```python
from build123d import *

# Parameters (mm, degrees)
BASE_EXTRUDE_THIN_DEPTH        = 19.05
CUT_EXTRUDE1_REACH             = 97.25
SKETCH2_R                      = 6.35
BOSS_EXTRUDE1_START            = -19.05
BOSS_EXTRUDE1_DEPTH            = 38.1
EXTRUDE_THIN1_DEPTH            = 38.1
CUT_EXTRUDE2_REACH             = 89.648
SKETCH4_W                      = 1.110971389
SKETCH4_H                      = 4.320444291
SKETCH4_W_2                    = 1.851618982
SKETCH4_H_2                    = 2.46882531
SKETCH4_W_3                    = 12.467567812
SKETCH4_H_3                    = 8.640888583
SKETCH4_W_4                    = 7.776799724
SKETCH4_H_4                    = 11.356596423
SKETCH4_W_5                    = 13.08477414
SKETCH4_H_5                    = 10.61594883
SKETCH4_W_6                    = 6.665828335
SKETCH4_H_6                    = 9.628418706
SKETCH4_W_7                    = 5.616577579
SKETCH4_H_7                    = 7.406475928
SKETCH4_W_8                    = 9.011212379
SKETCH4_H_8                    = 6.665828335
SKETCH4_W_9                    = 6.172063273
SKETCH4_H_9                    = 2.839149106
SKETCH4_W_10                   = 4.999371251
SKETCH4_H_10                   = 12.344126546
CUT_EXTRUDE2_DIRECTION_2_DEPTH = 55.324508946
FILLET1_R                      = 5.08


with BuildPart() as part:
    # Sketch1 → Base-Extrude-Thin (new body, symmetric)
    with BuildSketch(Plane(origin=(0, 0, 0), x_dir=(0, 0, -1), z_dir=(1, 0, 0))):
        with BuildLine():
            Line((-77.216478592, 27.494340102), (-45.335245167, 0.742808893))
            ThreePointArc((-45.335245167, 0.742808893), (-44.380308461, 0.191475929), (-43.294394506, 0))
            Line((-43.294394506, 0), (-3.175, 0))
            ThreePointArc((-3.175, 0), (-0.92993597, 0.92993597), (0, 3.175))
            Line((0, 3.175), (0, 79.375))
            ThreePointArc((0, 79.375), (-0.92993597, 81.62006403), (-3.175, 82.55))
            Line((-3.175, 82.55), (-57.15, 82.55))
            Line((-57.15, 82.55), (-57.15, 88.9))
            Line((-57.15, 88.9), (-3.175, 88.9))
            ThreePointArc((-3.175, 88.9), (3.560192091, 86.110192091), (6.35, 79.375))
            Line((6.35, 79.375), (6.35, 3.175))
            ThreePointArc((6.35, 3.175), (3.560192091, -3.560192091), (-3.175, -6.35))
            Line((-3.175, -6.35), (-43.294394506, -6.35))
            ThreePointArc((-43.294394506, -6.35), (-46.552136371, -5.775572213), (-49.416946488, -4.121573321))
            Line((-49.416946488, -4.121573321), (-81.298179914, 22.629957888))
            Line((-81.298179914, 22.629957888), (-77.216478592, 27.494340102))
        make_face()
    extrude(amount=BASE_EXTRUDE_THIN_DEPTH, both=True)

    # Sketch2 → Cut-Extrude1 (cut, up to next)
    with BuildSketch(Plane(origin=(0, 88.9, 0), x_dir=(-1, 0, 0), z_dir=(0, 1, 0)), mode=Mode.PRIVATE) as cut_extrude1_sk1:
        with Locations((0, 38.1)):
            Circle(SKETCH2_R)
    cut_extrude1_tool1 = extrude(cut_extrude1_sk1.sketch, amount=-CUT_EXTRUDE1_REACH, mode=Mode.PRIVATE) & part.part
    add(cut_extrude1_tool1.solids().sort_by_distance((0, 88.9, 38.1))[0], mode=Mode.SUBTRACT)

    # Sketch3 → Boss-Extrude1 (add)
    with BuildSketch(Plane(origin=(0, 0, 0), x_dir=(0, 0, -1), z_dir=(1, 0, 0)).offset(BOSS_EXTRUDE1_START)):
        with BuildLine():
            Line((-49.416946488, -4.121573321), (-81.298179914, 22.629957888))
            Line((-81.298179914, 22.629957888), (-81.298179914, -6.35))
            Line((-81.298179914, -6.35), (-43.294394506, -6.35))
            ThreePointArc((-43.294394506, -6.35), (-46.552136371, -5.775572213), (-49.416946488, -4.121573321))
        make_face()
    extrude(amount=BOSS_EXTRUDE1_DEPTH)

    # Sketch5 → Extrude-Thin1 (add, through all)
    with BuildSketch(Plane(origin=(19.05, 0, 0), x_dir=(0, 0, -1), z_dir=(1, 0, 0))):
        Polygon((-3.175, 88.9), (60.674508946, 88.9), (60.674508946, -6.35), (-3.175, -6.35), (-3.175, -1.27), (55.594508946, -1.27), (55.594508946, 83.82), (-3.175, 83.82), align=None)
    extrude(amount=-EXTRUDE_THIN1_DEPTH)

    # Sketch4 → Cut-Extrude2 (cut, up to next)
    with BuildSketch(Plane(origin=(0, 0, -6.35), x_dir=(-1, 0, 0), z_dir=(0, 0, -1)), mode=Mode.PRIVATE) as cut_extrude2_sk1:
        with Locations((-12.40584718, 74.110376614)):
            Rectangle(SKETCH4_W, SKETCH4_H)
    cut_extrude2_tool1 = extrude(cut_extrude2_sk1.sketch, amount=-CUT_EXTRUDE2_REACH, mode=Mode.PRIVATE) & part.part
    add(cut_extrude2_tool1.solids().sort_by_distance((12.405847, 74.110377, -6.35))[0], mode=Mode.SUBTRACT)
    # Sketch4 → Cut-Extrude2 (cut, up to next)
    with BuildSketch(Plane(origin=(0, 0, -6.35), x_dir=(-1, 0, 0), z_dir=(0, 0, -1)), mode=Mode.PRIVATE) as cut_extrude2_sk2:
        with Locations((-2.160222146, 58.001291471)):
            Rectangle(SKETCH4_W_2, SKETCH4_H_2)
    cut_extrude2_tool2 = extrude(cut_extrude2_sk2.sketch, amount=-CUT_EXTRUDE2_REACH, mode=Mode.PRIVATE) & part.part
    add(cut_extrude2_tool2.solids().sort_by_distance((2.160222, 58.001291, -6.35))[0], mode=Mode.SUBTRACT)
    # Sketch4 → Cut-Extrude2 (cut, up to next)
    with BuildSketch(Plane(origin=(0, 0, -6.35), x_dir=(-1, 0, 0), z_dir=(0, 0, -1)), mode=Mode.PRIVATE) as cut_extrude2_sk3:
        with Locations((-3.641517331, 41.336720633)):
            Rectangle(SKETCH4_W_3, SKETCH4_H_3)
    cut_extrude2_tool3 = extrude(cut_extrude2_sk3.sketch, amount=-CUT_EXTRUDE2_REACH, mode=Mode.PRIVATE) & part.part
    add(cut_extrude2_tool3.solids().sort_by_distance((3.641517, 41.336721, -6.35))[0], mode=Mode.SUBTRACT)
    # Sketch4 → Cut-Extrude2 (cut, up to next)
    with BuildSketch(Plane(origin=(0, 0, -6.35), x_dir=(-1, 0, 0), z_dir=(0, 0, -1)), mode=Mode.PRIVATE) as cut_extrude2_sk4:
        with Locations((10.183904401, 58.248174002)):
            Rectangle(SKETCH4_W_4, SKETCH4_H_4)
    cut_extrude2_tool4 = extrude(cut_extrude2_sk4.sketch, amount=-CUT_EXTRUDE2_REACH, mode=Mode.PRIVATE) & part.part
    add(cut_extrude2_tool4.solids().sort_by_distance((-10.183904, 58.248174, -6.35))[0], mode=Mode.SUBTRACT)
    # Sketch4 → Cut-Extrude2 (cut, up to next)
    with BuildSketch(Plane(origin=(0, 0, -6.35), x_dir=(-1, 0, 0), z_dir=(0, 0, -1)), mode=Mode.PRIVATE) as cut_extrude2_sk5:
        with Locations((-5.307974415, 22.326765751)):
            Rectangle(SKETCH4_W_5, SKETCH4_H_5)
    cut_extrude2_tool5 = extrude(cut_extrude2_sk5.sketch, amount=-CUT_EXTRUDE2_REACH, mode=Mode.PRIVATE) & part.part
    add(cut_extrude2_tool5.solids().sort_by_distance((5.307974, 22.326766, -6.35))[0], mode=Mode.SUBTRACT)
    # Sketch4 → Cut-Extrude2 (cut, up to next)
    with BuildSketch(Plane(origin=(0, 0, -6.35), x_dir=(-1, 0, 0), z_dir=(0, 0, -1)), mode=Mode.PRIVATE) as cut_extrude2_sk6:
        with Locations((9.628418706, 21.833000689)):
            Rectangle(SKETCH4_W_6, SKETCH4_H_6)
    cut_extrude2_tool6 = extrude(cut_extrude2_sk6.sketch, amount=-CUT_EXTRUDE2_REACH, mode=Mode.PRIVATE) & part.part
    add(cut_extrude2_tool6.solids().sort_by_distance((-9.628419, 21.833001, -6.35))[0], mode=Mode.SUBTRACT)
    # Sketch4 → Cut-Extrude2 (cut, up to next)
    with BuildSketch(Plane(origin=(0, 0, -6.35), x_dir=(-1, 0, 0), z_dir=(0, 0, -1)), mode=Mode.PRIVATE) as cut_extrude2_sk7:
        with Locations((7.375615612, 40.719514305)):
            Rectangle(SKETCH4_W_7, SKETCH4_H_7)
    cut_extrude2_tool7 = extrude(cut_extrude2_sk7.sketch, amount=-CUT_EXTRUDE2_REACH, mode=Mode.PRIVATE) & part.part
    add(cut_extrude2_tool7.solids().sort_by_distance((-7.375616, 40.719514, -6.35))[0], mode=Mode.SUBTRACT)
    # Sketch4 → Cut-Extrude2 (cut, up to next)
    with BuildSketch(Plane(origin=(0, 0, -6.35), x_dir=(-1, 0, 0), z_dir=(0, 0, -1)), mode=Mode.PRIVATE) as cut_extrude2_sk8:
        with Locations((-0.802368225, 69.728211691)):
            Rectangle(SKETCH4_W_8, SKETCH4_H_8)
    cut_extrude2_tool8 = extrude(cut_extrude2_sk8.sketch, amount=-CUT_EXTRUDE2_REACH, mode=Mode.PRIVATE) & part.part
    add(cut_extrude2_tool8.solids().sort_by_distance((0.802368, 69.728212, -6.35))[0], mode=Mode.SUBTRACT)
    # Sketch4 → Cut-Extrude2 (cut, up to next)
    with BuildSketch(Plane(origin=(0, 0, -6.35), x_dir=(-1, 0, 0), z_dir=(0, 0, -1)), mode=Mode.PRIVATE) as cut_extrude2_sk9:
        with Locations((-3.086031637, 49.17524099)):
            Rectangle(SKETCH4_W_9, SKETCH4_H_9)
    cut_extrude2_tool9 = extrude(cut_extrude2_sk9.sketch, amount=-CUT_EXTRUDE2_REACH, mode=Mode.PRIVATE) & part.part
    add(cut_extrude2_tool9.solids().sort_by_distance((3.086032, 49.175241, -6.35))[0], mode=Mode.SUBTRACT)
    # Sketch4 → Cut-Extrude2 (cut, up to next)
    with BuildSketch(Plane(origin=(0, 0, -6.35), x_dir=(-1, 0, 0), z_dir=(0, 0, -1)), mode=Mode.PRIVATE) as cut_extrude2_sk10:
        with Locations((-9.906161554, 57.75440894)):
            Rectangle(SKETCH4_W_10, SKETCH4_H_10)
    cut_extrude2_tool10 = extrude(cut_extrude2_sk10.sketch, amount=-CUT_EXTRUDE2_REACH, mode=Mode.PRIVATE) & part.part
    add(cut_extrude2_tool10.solids().sort_by_distance((9.906162, 57.754409, -6.35))[0], mode=Mode.SUBTRACT)

    # Sketch4 → Cut-Extrude2 direction 2 (cut)
    with BuildSketch(Plane(origin=(0, 0, -6.35), x_dir=(-1, 0, 0), z_dir=(0, 0, -1))):
        with Locations((-12.40584718, 74.110376614)):
            Rectangle(SKETCH4_W, SKETCH4_H)
        with Locations((-2.160222146, 58.001291471)):
            Rectangle(SKETCH4_W_2, SKETCH4_H_2)
        with Locations((-3.641517331, 41.336720633)):
            Rectangle(SKETCH4_W_3, SKETCH4_H_3)
        with Locations((10.183904401, 58.248174002)):
            Rectangle(SKETCH4_W_4, SKETCH4_H_4)
        with Locations((-5.307974415, 22.326765751)):
            Rectangle(SKETCH4_W_5, SKETCH4_H_5)
        with Locations((9.628418706, 21.833000689)):
            Rectangle(SKETCH4_W_6, SKETCH4_H_6)
        with Locations((7.375615612, 40.719514305)):
            Rectangle(SKETCH4_W_7, SKETCH4_H_7)
        with Locations((-0.802368225, 69.728211691)):
            Rectangle(SKETCH4_W_8, SKETCH4_H_8)
        with Locations((-3.086031637, 49.17524099)):
            Rectangle(SKETCH4_W_9, SKETCH4_H_9)
        with Locations((-9.906161554, 57.75440894)):
            Rectangle(SKETCH4_W_10, SKETCH4_H_10)
    extrude(amount=CUT_EXTRUDE2_DIRECTION_2_DEPTH, mode=Mode.SUBTRACT)

    # Fillet1
    fillet1_edges = [part.edges().sort_by_distance(p)[0] for p in [
        (0, 88.9, -60.674508946),
        (0, -6.35, -60.674508946),
    ]]
    fillet(fillet1_edges, radius=FILLET1_R)


solid = part.part
```
The model under review builds one solid part; all positions refer to its coordinate system, in mm. A direction names the side the tool comes from. Give positions to 0.01 mm unless a question says otherwise; leave off trailing zeros. Write each loop counter-clockwise with the first axis right and the second up, starting at its lowest first coordinate (ties: lowest second). Pieces come first, ordered by that corner, then holes.
(1) Consider section D-D, the plane y = 15.5. Give the boundary of the cut face in (x, z).
(2) To check wall thickness, follow L1, parallel to X at y = 85, z = 38; L2, parallel to X at y = 72.5, z = -6; L3, parallel to Z at x = 17.5, y = 63.5. State the ranges of each line that lie inside material, in increasing order.
(3) The part is to be moulded in two halves that separate along X. For faces 1 (the flat face through (-7, 37.016, -58)), 2 (the cylindrical face through (-0.27, 87.45, -59.15)), say which applies: released by +X, released by -X, zero draft, split by the parting line, or undercut.
(4) Consider section C-C, the plane z = 38.1. Give the boundary of the cut face in (x, y), and give its area (3 significant figures).
(5) For P1, Ø1.5, axis at x = 7, z = -57, coming from the -Y side; P2, Ø0.6, axis at x = 12.5, z = -57.5, coming from the -Y side; P3, Ø5, axis at x = 5, y = 74, coming from the +Z side, all flat-tipped, find the tip position at first contact; note any pin that passes through.
(6) Tool access review of faces 3 (the flat face through (-10, 17.019, -58)), 4 (the flat face through (0, 83.82, -31)), 5 (the flat face through (-10, 63.926, -58)), 6 (the flat face through (0, 88.9, 2)): name each direction out of +Z, -Z, +X, -X, +Y, -Y from which nothing blocks a thin tool from reaching the whole face with its end or side.
(7) Consider section A-A, the plane z = -40.5. Give the boundary of the cut face in (x, y), and give its area (3 significant figures).
(8) Consider section B-B, the plane y = 40. Give the boundary of the cut face in (x, z), and give its area (3 significant figures).
Returned:
1. outline: (-19.05, -60.67) - (19.05, -60.67) - (19.05, -55.59) - (-19.05, -55.59) - close; (-19.05, -6.35) - (19.05, -6.35) - (19.05, 0) - (-19.05, 0) - close; (-19.05, 62.92) - (19.05, 62.92) - (19.05, 81.3) - (-19.05, 81.3) - close
2. L1: x = -19.05 to -6.35, 6.35 to 19.05
2. L2: x = -19.05 to -3.7, 5.31 to 11.85, 12.96 to 19.05
2. L3: z = -60.67 to -55.59, -6.35 to 0
3. face 1: undercut
3. face 2: zero draft
4. outline: (-19.05, -6.35) - (19.05, -6.35) - (19.05, 0) - (-19.05, 0) - close; (-19.05, 82.55) - (-6.35, 82.55) - (-6.35, 88.9) - (-19.05, 88.9) - close; (6.35, 82.55) - (19.05, 82.55) - (19.05, 88.9) - (6.35, 88.9) - close
4. area: 403 mm2
5. P1: stops at y = -6.31
5. P2: stops at y = -6.09
5. P3: stops at z = 0
6. face 3: -Z
6. face 4: +X, -X
6. face 5: +Z, -Z
6. face 6: +Z, -Z, +X, -X, +Y
7. outline: (-19.05, -6.35) - (19.05, -6.35) - (19.05, -1.27) - (-19.05, -1.27) - close; (-19.05, 83.82) - (19.05, 83.82) - (19.05, 88.9) - (-19.05, 88.9) - close
7. area: 387 mm2
8. outline: (-19.05, -60.67) - (-10.18, -60.67) - (-10.18, -55.59) - (-19.05, -55.59) - close; (-19.05, -6.35) - (-10.18, -6.35) - (-10.18, 0) - (-19.05, 0) - close; (-4.57, -60.67) - (-2.59, -60.67) - (-2.59, -55.59) - (-4.57, -55.59) - close; (-4.57, -6.35) - (-2.59, -6.35) - (-2.59, 0) - (-4.57, 0) - close; (9.88, -60.67) - (19.05, -60.67) - (19.05, -55.59) - (9.88, -55.59) - close; (9.88, -6.35) - (19.05, -6.35) - (19.05, 0) - (9.88, 0) - close
8. area: 229 mm2
